Input: dimensioned drawing with shaded views. Units: mm. Origin: part minimum x, y, z. A direction names the side the tool comes from. Coordinates: 2 decimals unless noted, no trailing zeros. Loops run counter-clockwise (first coordinate to the right, second up) from the corner with the lowest first, then second, coordinate; pieces in that order, holes last.
Item 1: Section A-A on z = 49.5. Return loops of the section in (x, y) (1 decimal).
Item 2: Section B-B on y = 40.5. Return loops of the section in (x, z), and give its area (3 significant figures).
Item 3: Section D-D on y = 6. Return loops of the section in (x, z) (1 decimal), and give its area (3 significant figures).
Item 4: Contact query for flat-ended pins moving along their axis: P1, Ø5, axis at x = 28.5, z = 47, coming from the -Y side; P2, Ø5.5, axis at x = 18, z = 47, coming from the -Y side (1 decimal); P3, Ø8, axis at x = 44, z = 8, coming from the +Y side; P4, Ø13.5, axis at x = 14, y = 8, coming from the -Z side. Output: stop coordinate, or through.
Item 5: Section C-C on x = 46.5. Return loops of the section in (y, z) (1 decimal).
Item 6: Reachability of the marked faces 5, 6, 7 and 8 from +Z, -Z, +X, -X, +Y, -Y: full face, straight path, thin tool, end or side. Return the list, or none.
Item 7: Ray query, line 1 along X through (y, z) = (42.5, 46); line 2 along Y through (x, z) = (40, 11.5) (1 decimal); line 3 along X through (y, z) = (24, 40). Return the intervals inside material, ascending.
Item 8: Pull-direction query (Y, two-part tool) for the marked faces 1, 2, 3 and 4; classes: released by +Y, released by -Y, zero draft, split by the parting line, or undercut.
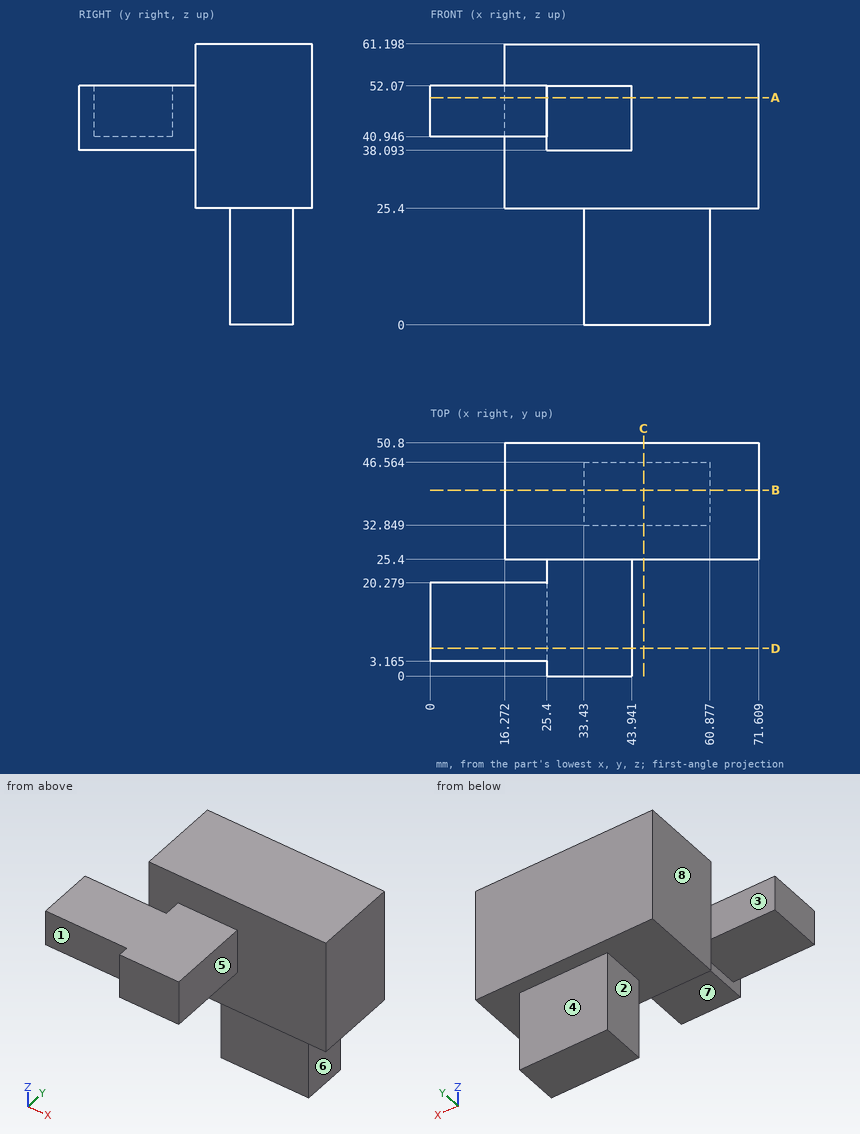
Results found:
1. outline: (0, 3.2) - (25.4, 3.2) - (25.4, 0) - (43.9, 0) - (43.9, 25.4) - (71.6, 25.4) - (71.6, 50.8) - (16.3, 50.8) - (16.3, 25.4) - (25.4, 25.4) - (25.4, 20.3) - (0, 20.3) - close
2. outline: (16.27, 25.4) - (33.43, 25.4) - (33.43, 0) - (60.88, 0) - (60.88, 25.4) - (71.61, 25.4) - (71.61, 61.2) - (16.27, 61.2) - close
2. area: 2,680 mm2
3. outline: (0, 40.9) - (25.4, 40.9) - (25.4, 38.1) - (43.9, 38.1) - (43.9, 52.1) - (0, 52.1) - close
3. area: 542 mm2
4. P1: stops at y = 0
4. P2: stops at y = 3.2
4. P3: stops at y = 46.56
4. P4: stops at z = 40.95
5. outline: (25.4, 25.4) - (32.8, 25.4) - (32.8, 0) - (46.6, 0) - (46.6, 25.4) - (50.8, 25.4) - (50.8, 61.2) - (25.4, 61.2) - close
6. face 5: +Z, -Z, +X, -Y
6. face 6: -Z, +X, +Y, -Y
6. face 7: -Z, +X, -X, -Y
6. face 8: +Z, -Z, -X, +Y
7. line 1: x = 16.27 to 71.61
7. line 2: y = 32.8 to 46.6
7. line 3: x = 25.4 to 43.94
8. face 1: released by -Y
8. face 2: zero draft
8. face 3: undercut
8. face 4: released by +Y
